Design review of the part shown in the three views and the two pictorial views. Dimensions are in mm from the part's minimum x, y and z. A direction names the side the tool comes from. Round coordinates to 2 decimals unless told otherwise and drop trailing zeros. Write each loop counter-clockwise with the first axis right and the second up, starting at its lowest first coordinate (ties: lowest second). Pieces come first, ordered by that corner, then holes. Notation, with made-up numbers: (-6, 27) -> (11, 27) arc R24 ccw to (11, 51) -> close; hole circle Ø9 at (-34, -36.75). An arc over 180 degrees is marked (long way). One line per question, with ' | ' between items. Start each with the question number.
1) Consider section A-A (y = 4.15). Give the boundary of the cut face in (x, z), then the cut area to 3 significant figures.
2) Consider section B-B (x = 17). Give the boundary of the cut face in (y, z), then the cut area to 3 significant figures.
3) Insertion check: pin 1 Ø2 at (x, y) = (17.5, 2) entering from +Z; pin 2 Ø2 at (x, z) = (17, 10) entering from -Y. Each pin has a flat end and moves straight along its axis. Give the tip position at first contact, or say it passes through.
4) Consider section D-D (y = 0.75). Give the boundary of the cut face in (x, z), then the cut area to 3 significant figures.
5) Consider section C-C (z = 7.5). Give the boundary of the cut face in (x, y), then the cut area to 3 significant figures.
6) Mouldability with a two-part tool opening along X and no side actions: class the marked faces 3, 4 and 5 as +X half, -X half, draft (parallel to the pull), parting line (faces both ways), or undercut.
7) For probe 1 along X at (y, z) = (0.7, 10.5) (1 decimal); probe 2 along Z at (x, y) = (10, 1.55); probe 3 along Z at (x, y) = (12, 0.4), list the stretches that pass through material, from the lowest coordinate up.
8) For the marked faces 1 and 2, list the 3-axis set-ups (+Z, -Z, +X, -X, +Y, -Y) from which the entire face can be reached by the end or side of a thin tool; tool diameter is ignored.
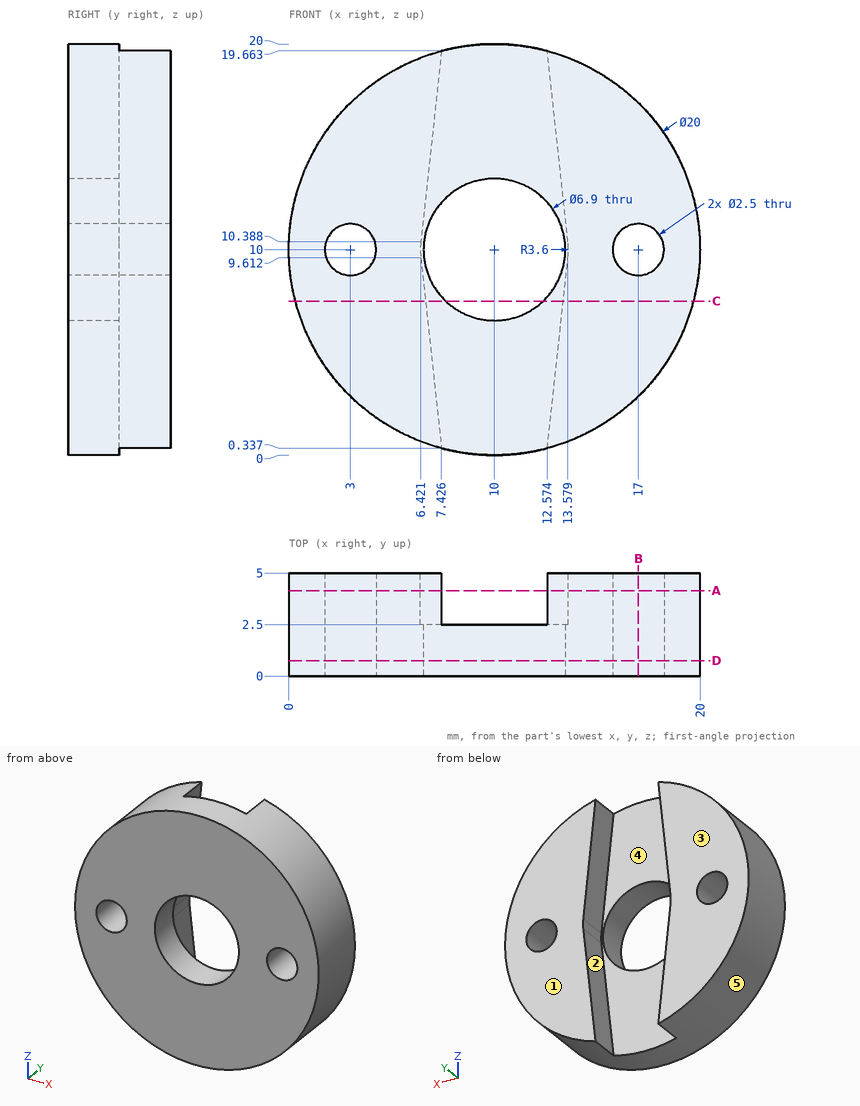
From the geometry:
1) outline: (6.42, 9.61) arc R3.6 cw to (6.42, 10.39) -> (7.43, 19.66) arc R10 ccw to (7.43, 0.34) -> close; (12.57, 0.34) arc R10 ccw to (12.57, 19.66) -> (13.58, 10.39) arc R3.6 cw to (13.58, 9.61) -> close; hole circle Ø2.5 at (3, 10); hole circle Ø2.5 at (17, 10) | area: 182 mm2
2) outline: (0, 2.86) -> (5, 2.86) -> (5, 8.75) -> (0, 8.75) -> close; (0, 11.25) -> (5, 11.25) -> (5, 17.14) -> (0, 17.14) -> close | area: 58.9 mm2
3) pin 1: stops at z = 17.6 | pin 2: passes through
4) outline: circle Ø20 at (10, 10); hole circle Ø2.5 at (3, 10); hole circle Ø6.9 at (10, 10); hole circle Ø2.5 at (17, 10) | area: 267 mm2
5) outline: (0.32, 0) -> (7.62, 0) -> (7.62, 2.5) -> (6.65, 2.5) -> (6.65, 5) -> (0.32, 5) -> close; (12.38, 0) -> (19.68, 0) -> (19.68, 5) -> (13.35, 5) -> (13.35, 2.5) -> (12.38, 2.5) -> close | area: 68.2 mm2
6) face 3: draft | face 4: undercut | face 5: parting line
7) probe 1: x = 0 to 1.9, 4.1 to 6.6, 13.4 to 15.9, 18.1 to 20 | probe 2: z = 0 to 6.55, 13.45 to 20 | probe 3: z = 0.2 to 7.19, 12.81 to 19.8
8) face 1: +Z, -Z, +X, -X, +Y | face 2: +Y
